Autodesk Inventor part; units mm, degrees
ref_plane "YZ Plane" through (0, 0, 0) normal (1, 0, 0) x (0, 1, 0)
ref_plane "XZ Plane" through (0, 0, 0) normal (0, 1, 0) x (-1, 0, 0)
ref_plane "XY Plane" through (0, 0, 0) normal (0, 0, 1) x (1, 0, 0)
sketch "podstawa" plane through (0, 0, 0) normal (0, 0, 1) x (1, 0, 0)
  line L0 (-30, -25) -> (30, -25)
  line L1 (30, -25) -> (30, 25)
  line L2 (30, 25) -> (-30, 25)
  line L3 (-30, 25) -> (-30, -25)
  circle A0 centre (0, 0) radius 5
  line L4 (0, 0) -> (24, 0) construction
  line L5 (24, 0) -> (24, 19) construction
  circle A1 centre (24, 19) radius 3
  line L6 (0, 25) -> (0, -25) construction
  circle A2 centre (-24, 19) radius 3
  line L7 (-30, 0) -> (30, 0) construction
  circle A3 centre (24, -19) radius 3
  circle A4 centre (-24, -19) radius 3
  dimension "d0" = 60
  dimension "d1" = 50
  dimension "d9" = 10
  dimension "d26" = 24
  dimension "d27" = 19
  dimension "d28" = 6
extrude "Wyciągnięcie proste1" add sketch "podstawa" along normal blind 8 contours L3 L2 L1 L0 | A1 | A2 | A3 | A4
sketch "nakladka" plane through (0, 0, 8) normal (0, 0, 1) x (1, 0, 0)
  line L0 (18, -25) -> (-18, -25)
  line L1 (-18, -25) -> (-18, 25)
  line L2 (-18, 25) -> (18, 25)
  line L3 (18, 25) -> (18, -25)
  line L4 (18, -25) -> (-18, 25) construction
  line L5 (-18, -25) -> (18, 25) construction
  line L6 (-9, -9) -> (9, -9)
  line L7 (9, -9) -> (9, 9)
  line L8 (9, 9) -> (-9, 9)
  line L9 (-9, 9) -> (-9, -9)
  line L10 (-9, -9) -> (9, 9) construction
  line L11 (9, -9) -> (-9, 9) construction
  point P0 (0, 0)
  dimension "d12" = 36
  dimension "d13" = 50
  dimension "d14" = 18
  dimension "d15" = 18
extrude "Wyciągnięcie proste2" add sketch "nakladka" along normal blind 12
sketch "srodek_2mm" plane through (0, 0, 8) normal (0, 0, 1) x (1, 0, 0)
  line L0 (-9, -9) -> (9, -9)
  line L1 (9, -9) -> (9, 9)
  line L2 (9, 9) -> (-9, 9)
  line L3 (-9, 9) -> (-9, -9)
  line L4 (-9, -9) -> (9, 9) construction
  line L5 (9, -9) -> (-9, 9) construction
  circle A0 centre (0, 0) radius 5
extrude "Wyciągnięcie proste3" add sketch "srodek_2mm" along normal blind 2
sketch "wyciecie_gora_6mm" plane through (0, 0, 20) normal (0, 0, 1) x (1, 0, 0)
  line L0 (-14, -4) -> (14, -4)
  line L1 (14, -4) -> (14, 4)
  line L2 (14, 4) -> (-14, 4)
  line L3 (-14, 4) -> (-14, -4)
  line L4 (-14, -4) -> (14, 4) construction
  line L5 (14, -4) -> (-14, 4) construction
  point P0 (0, 0)
  dimension "d20" = 28
  dimension "d21" = 8
extrude "Wyciągnięcie proste4" cut sketch "wyciecie_gora_6mm" against normal blind 6
extrude "Wyciągnięcie proste5" cut sketch "podstawa" along normal through all contours A1 | A2 | A3 | A4
properties part number "Bartosz_Zukowski_model_nr_7"
For this review, take the finished solid that the model builds, in its own axes (mm). A direction names the side the tool comes from. Give positions to 0.01 mm unless a question says otherwise; leave off trailing zeros. Loops run counter-clockwise (first coordinate to the right, second up) from the corner with the lowest first, then second, coordinate; pieces in that order, holes last. Notation, with made-up numbers: M 35.25,26 L 60.25,26 A17 ccw 60.25,36 Z; hole C 35.5,41.5 d3. An arc over 180 degrees is marked long. Answer as a JSON object with one key per item and string values. Group by question number.
Q1. Insertion check: P1, Ø6.5, axis at y = 0, z = 18.5, coming from the +X side; P2, Ø7, axis at x = -24, y = 19, coming from the +Z side; P3, Ø12, axis at y = -13.5, z = 14.5, coming from the -X side. Each pin has a flat end and moves straight along its axis. Give the tip position at first contact, or say it passes through.
Q2. For probe 1 along Y at (x, z) = (-24, 2); probe 2 along X at (y, z) = (-19, 5); probe 3 along X at (y, z) = (4, 12.5), list the stretches that pass through material, from the lowest coordinate up. Write a range as [from, to].
Q3. Mouldability with a two-part tool opening along X and no side actions: class faces 4 (the flat face through (11, 0, 14)), 5 (the flat face through (0, 25, 8)), 6 (the flat face through (-30, 0, 4)) as +X half, -X half, draft (parallel to the pull), parting line (faces both ways), or undercut.
Q4. Add section A-A on y = 0. Give the boundary of the cut face in (x, z), and give its area (3 significant figures).
Q5. Add section C-C on y = -19. Give the boundary of the cut face in (x, z), and give its area (3 significant figures).
Q6. Tool access review of faces 1 (the flat face through (18, 0, 14)), 2 (the flat face through (-24, 0, 8)), 3 (the flat face through (-9, 0.1, 13.8)): name each direction out of +Z, -Z, +X, -X, +Y, -Y from which nothing blocks a thin tool from reaching the whole face with its end or side.
Q7. Add section B-B on x = 0. Give the boundary of the cut face in (y, z), and give its area (3 significant figures).
Q8. Add section D-D on z = 1.5. Give the boundary of the cut face in (x, y), and give its area (3 significant figures).
Checked values:
{
 "1": {"P1": "x = 18", "P2": "z = 8", "P3": "x = -18"},
 "2": {"probe 1": "[-25, -22], [-16, 16], [22, 25]", "probe 2": "[-30, -27], [-21, 21], [27, 30]", "probe 3": "[-18, -9], [9, 18]"},
 "3": {"face 4": "undercut", "face 5": "draft", "face 6": "-X half"},
 "4": {"outline": "M -30,0 L -5,0 L -5,10 L -9,10 L -9,14 L -14,14 L -14,20 L -18,20 L -18,8 L -30,8 Z; M 5,0 L 30,0 L 30,8 L 18,8 L 18,20 L 14,20 L 14,14 L 9,14 L 9,10 L 5,10 Z", "area": "572 mm²"},
 "5": {"outline": "M -30,0 L -27,0 L -27,8 L -30,8 Z; M -21,0 L 21,0 L 21,8 L 18,8 L 18,20 L -18,20 L -18,8 L -21,8 Z; M 27,0 L 30,0 L 30,8 L 27,8 Z", "area": "816 mm²"},
 "6": {"face 1": "+Z, +X, +Y, -Y", "face 2": "+Z, -X, +Y, -Y", "face 3": "+Z"},
 "7": {"outline": "M -25,0 L -5,0 L -5,10 L -9,10 L -9,20 L -25,20 Z; M 5,0 L 25,0 L 25,20 L 9,20 L 9,10 L 5,10 Z", "area": "720 mm²"},
 "8": {"outline": "M -30,-25 L 30,-25 L 30,25 L -30,25 Z; hole C -24,-19 d6; hole C -24,19 d6; hole C 0,0 d10; hole C 24,-19 d6; hole C 24,19 d6", "area": "2,810 mm²"}
}
